from build123d import *

# Parameters (mm, degrees)
CYLINDER323_R               = 1.5
CYLINDER323_DEPTH           = 30
CYLINDER323_PLACEMENT_ANGLE = 67.5
CYLINDER324_R               = 1.5
CYLINDER324_DEPTH           = 30
CYLINDER324_PLACEMENT_ANGLE = 112.5
CYLINDER011_R               = 1.5
CYLINDER011_DEPTH           = 30
CYLINDER011_PLACEMENT_ANGLE = 157.5
CYLINDER012_R               = 1.5
CYLINDER012_DEPTH           = 30
CYLINDER012_PLACEMENT_ANGLE = 202.5
CYLINDER013_R               = 1.5
CYLINDER013_DEPTH           = 30
CYLINDER013_PLACEMENT_ANGLE = 112.500002
CYLINDER014_R               = 1.5
CYLINDER014_DEPTH           = 30
CYLINDER014_PLACEMENT_ANGLE = 67.5
CYLINDER015_R               = 1.5
CYLINDER015_DEPTH           = 30
CYLINDER015_PLACEMENT_ANGLE = 22.5
CYLINDER325_R               = 1.5
CYLINDER325_DEPTH           = 30
CYLINDER325_PLACEMENT_ANGLE = 22.5
TUBE004_R                   = 46
TUBE004_R_2                 = 38
TUBE004_DEPTH               = 1


with BuildPart() as obj1:
    # Cylinder323 → Cylinder323 (new body)
    with BuildSketch(Plane.XY):
        Circle(CYLINDER323_R)
    extrude(amount=CYLINDER323_DEPTH)


with BuildPart() as obj1_1:
    # Cylinder323 placement: moved
    add(obj1.part.moved(Location((-16.072704, -38.80294, 40))).rotate(Axis((-16.072704, -38.80294, 40), (0, 0, 1)), CYLINDER323_PLACEMENT_ANGLE))


with BuildPart() as obj2:
    # Cylinder324 → Cylinder324 (new body)
    with BuildSketch(Plane.XY):
        Circle(CYLINDER324_R)
    extrude(amount=CYLINDER324_DEPTH)


with BuildPart() as obj2_1:
    # Cylinder324 placement: moved
    add(obj2.part.moved(Location((16.072704, -38.80294, 40))).rotate(Axis((16.072704, -38.80294, 40), (0, 0, 1)), CYLINDER324_PLACEMENT_ANGLE))


with BuildPart() as obj3:
    # Cylinder011 → Cylinder011 (new body)
    with BuildSketch(Plane.XY):
        Circle(CYLINDER011_R)
    extrude(amount=CYLINDER011_DEPTH)


with BuildPart() as obj3_1:
    # Cylinder011 placement: moved
    add(obj3.part.moved(Location((38.80294, -16.072704, 40))).rotate(Axis((38.80294, -16.072704, 40), (0, 0, 1)), CYLINDER011_PLACEMENT_ANGLE))


with BuildPart() as obj4:
    # Cylinder012 → Cylinder012 (new body)
    with BuildSketch(Plane.XY):
        Circle(CYLINDER012_R)
    extrude(amount=CYLINDER012_DEPTH)


with BuildPart() as obj4_1:
    # Cylinder012 placement: moved
    add(obj4.part.moved(Location((38.80294, 16.072704, 40))).rotate(Axis((38.80294, 16.072704, 40), (0, 0, 1)), CYLINDER012_PLACEMENT_ANGLE))


with BuildPart() as obj5:
    # Cylinder013 → Cylinder013 (new body)
    with BuildSketch(Plane.XY):
        Circle(CYLINDER013_R)
    extrude(amount=CYLINDER013_DEPTH)


with BuildPart() as obj5_1:
    # Cylinder013 placement: moved
    add(obj5.part.moved(Location((16.072704, 38.80294, 40))).rotate(Axis((16.072704, 38.80294, 40), (0, 0, -1)), CYLINDER013_PLACEMENT_ANGLE))


with BuildPart() as obj6:
    # Cylinder014 → Cylinder014 (new body)
    with BuildSketch(Plane.XY):
        Circle(CYLINDER014_R)
    extrude(amount=CYLINDER014_DEPTH)


with BuildPart() as obj6_1:
    # Cylinder014 placement: moved
    add(obj6.part.moved(Location((-16.072704, 38.80294, 40))).rotate(Axis((-16.072704, 38.80294, 40), (0, 0, -1)), CYLINDER014_PLACEMENT_ANGLE))


with BuildPart() as obj7:
    # Cylinder015 → Cylinder015 (new body)
    with BuildSketch(Plane.XY):
        Circle(CYLINDER015_R)
    extrude(amount=CYLINDER015_DEPTH)


with BuildPart() as obj7_1:
    # Cylinder015 placement: moved
    add(obj7.part.moved(Location((-38.80294, 16.072704, 40))).rotate(Axis((-38.80294, 16.072704, 40), (0, 0, -1)), CYLINDER015_PLACEMENT_ANGLE))


with BuildPart() as compound249:
    # Cylinder325 → Cylinder325 (new body)
    with BuildSketch(Plane.XY):
        Circle(CYLINDER325_R)
    extrude(amount=CYLINDER325_DEPTH)


with BuildPart() as compound249_1:
    # Cylinder325 placement: moved
    add(compound249.part.moved(Location((-38.80294, -16.072704, 40))).rotate(Axis((-38.80294, -16.072704, 40), (0, 0, 1)), CYLINDER325_PLACEMENT_ANGLE))

    # Compound249: union obj1, obj2, obj3, obj4, obj5, obj6, obj7
    add(obj1_1.part)
    add(obj2_1.part)
    add(obj3_1.part)
    add(obj4_1.part)
    add(obj5_1.part)
    add(obj6_1.part)
    add(obj7_1.part)


with BuildPart() as obj8:
    # Tube004 → Tube004 (new body)
    with BuildSketch(Plane.XY.offset(50)):
        Circle(TUBE004_R)
        Circle(TUBE004_R_2, mode=Mode.SUBTRACT)
    extrude(amount=TUBE004_DEPTH)

    # Cut011: cut Compound249
    add(compound249_1.part, mode=Mode.SUBTRACT)


with BuildPart() as obj8_1:
    # Cut011 placement: moved
    add(obj8.part.moved(Location((0, 0, -61))))


solid = obj8_1.part
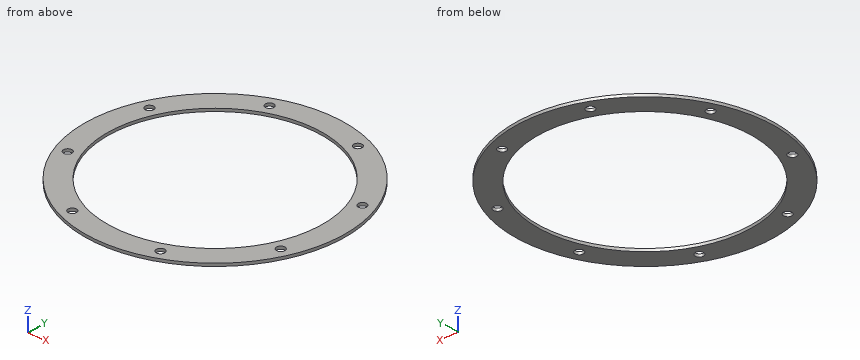
CAD build for the part. Positions are in the model's coordinates, mm. Give positions to 0.01 mm unless a question says otherwise; leave off trailing zeros. Write each loop counter-clockwise with the first axis right and the second up, starting at its lowest first coordinate (ties: lowest second). Pieces come first, ordered by that corner, then holes. Notation, with made-up numbers: (51.5, 14) - (93.5, 14) arc R9 ccw to (93.5, 31) - close; hole circle Ø3 at (49.5, 11). An arc over 180 degrees is marked (long way). Put each result on its own line as item: value.
(1) Wall check: L1, parallel to X at y = -17, z = -10.15; L2, parallel to Y at x = -1, z = -10.05; L3, parallel to X at y = -16.5, z = -10.65. Give the ranges that are in metal, low to high.
Working result:
L1: -42.74 to -39.98, -37.62 to -33.99, 33.99 to 37.62, 39.98 to 42.74
L2: -45.99 to -37.99, 37.99 to 45.99
L3: -42.94 to -40.24, -37.37 to -34.23, 34.23 to 37.37, 40.24 to 42.94
(2) Saw through at A-A (x = 0). List the corners of the cut face in (y, z), then the cut area to 3 significant figures.
Working result:
outline: (-46, -11) - (-38, -11) - (-38, -10) - (-46, -10) - close; (38, -11) - (46, -11) - (46, -10) - (38, -10) - close
area: 16.0 mm^2
(3) Saw through at C-C (z = -10.45). Count the separate pieces of the cut face and the enclosed holes in it, then the cut area to 3 significant figures.
Working result:
separate pieces: 1
enclosed holes: 9
area: 2,050 mm^2
